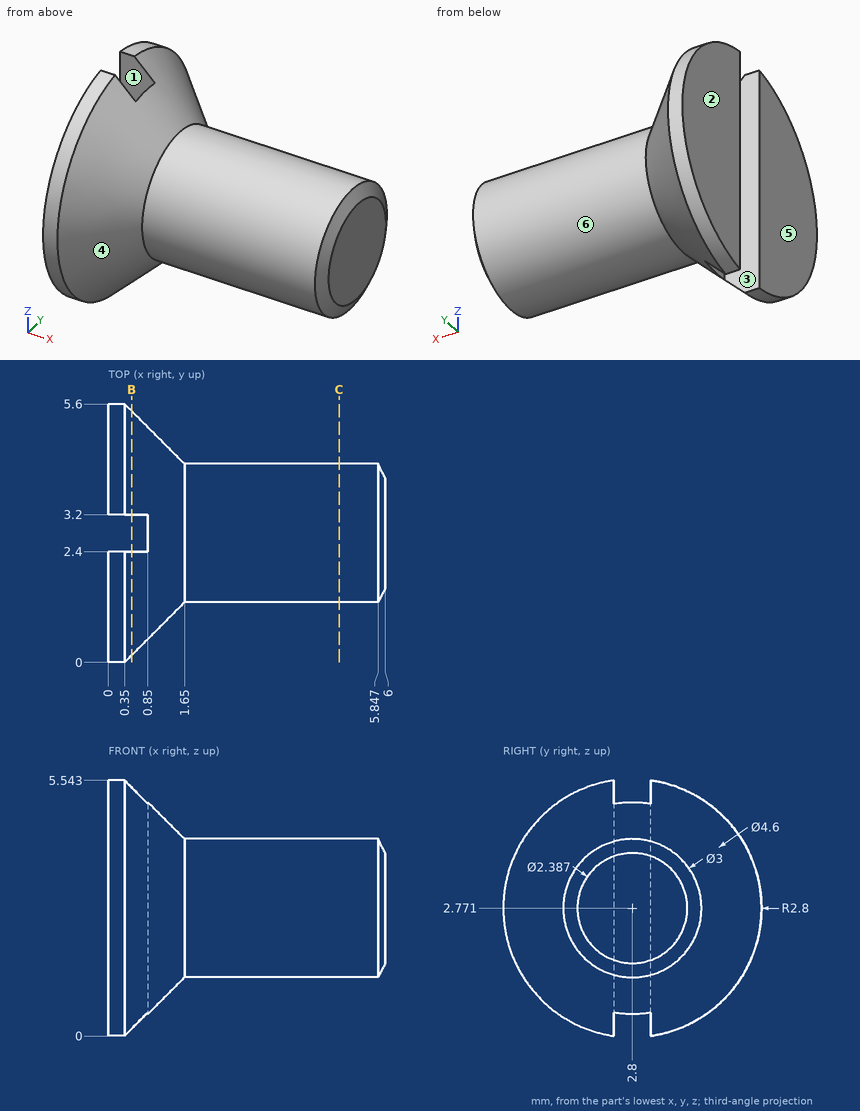
Can you work these out from the drawing? Everything is in mm from the part's minimum corner. A direction names the side the tool comes from. Coordinates: 2 decimals unless noted, no trailing zeros. Write each loop counter-clockwise with the first axis right and the second up, starting at its lowest first coordinate (ties: lowest second). Pieces come first, ordered by that corner, then holes. Notation, with made-up numbers: (14.25, 47) -> (29.25, 47) arc R13 ccw to (29.25, 57) -> close; hole circle Ø9 at (57.5, 84). An arc over 180 degrees is marked (long way). Write item = value, one per line.
(1) If I drill on probe 1 along Z at (x, y) = (4.25, 2.75); probe 2 along X at (y, z) = (2.65, 3.85); probe 3 along Y at (x, z) = (0.75, 0.75) (1 decimal), over which ranges is the centre line in solid material (lowest first)?
Verdict:
probe_1 = 1.27 to 4.27
probe_2 = 0.85 to 6
probe_3 = 1.5 to 2.4, 3.2 to 4.1
(2) On a 3-axis mill with a long thin cutter (end or side, diameter ignored), from which of +Z, -Z, +X, -X, +Y, -Y can I reach the whole of each face in a straight line? I mean the marked faces 5 and 6. Say none if no direction works.
Verdict:
face_5 = +Z, -Z, -X, +Y, -Y
face_6 = +X
(3) Thinking about a two-plate mould opening in Y: for the marked faces 1, 2, 3 and 4, which applies, +Y half, -Y half, draft (parallel to the pull), parting line (faces both ways), or undercut?
Verdict:
face_1 = undercut
face_2 = draft
face_3 = undercut
face_4 = parting line
(4) Imagine slicing it at B-B (x = 0.5). Please give me the cut outline in (y, z).
Verdict:
outline = (2.4, 0.15) -> (2.4, 5.39) arc R2.65 ccw to start; (3.2, 0.15) arc R2.65 ccw to (3.2, 5.39) -> close
(5) For pin 1 (1 mm diameter, centred on x = 1.5, z = 2, fed in from -Y) (1 decimal); pin 2 (1 mm diameter, centred on y = 4.5, z = 2.5, fed in from +X) (1 decimal), each with a flat end and sliding along its axis, tell me the tip position at first contact or that it passes through.
Verdict:
pin_1 = 0.8
pin_2 = 6
(6) Imagine slicing it at C-C (x = 5). Please give me the cut outline in (y, z).
Verdict:
outline = circle Ø3 at (2.8, 2.77)
